from build123d import *

# Parameters (mm, degrees)
SKETCH1_R           = 2.5
SKETCH1_R_2         = 10.25
BOSS_EXTRUDE1_DEPTH = 5


with BuildPart() as part:
    # Sketch1 → Boss-Extrude1 (new body)
    with BuildSketch(Plane.XY):
        with BuildLine():
            Line((-18.262940366, -7.217732658), (-10.073546599, -13.382307683))
            ThreePointArc((-10.073546599, -13.382307683), (0, -16.75), (10.073546599, -13.382307683))
            Line((10.073546599, -13.382307683), (18.262940366, -7.217732658))
            ThreePointArc((18.262940366, -7.217732658), (21.863878029, 0), (18.262940366, 7.217732658))
            Line((18.262940366, 7.217732658), (10.073546599, 13.382307683))
            ThreePointArc((10.073546599, 13.382307683), (0, 16.75), (-10.073546599, 13.382307683))
            Line((-10.073546599, 13.382307683), (-18.262940366, 7.217732658))
            ThreePointArc((-18.262940366, 7.217732658), (-21.863878029, 0), (-18.262940366, -7.217732658))
        make_face()
        with Locations((14.5, 0)):
            Circle(SKETCH1_R, mode=Mode.SUBTRACT)
        with Locations((-14.5, 0)):
            Circle(SKETCH1_R, mode=Mode.SUBTRACT)
        Circle(SKETCH1_R_2, mode=Mode.SUBTRACT)
    extrude(amount=BOSS_EXTRUDE1_DEPTH)


solid = part.part
Verification items for the finished model (mm, model axes). Coordinates: 2 decimals unless noted, no trailing zeros. Write each loop counter-clockwise with the first axis right and the second up, starting at its lowest first coordinate (ties: lowest second). Pieces come first, ordered by that corner, then holes. Notation, with made-up numbers: (81, 15.5) - (140, 15.5) arc R23 cw to (140, 54.5) - close; hole circle Ø10 at (82, 37). An arc over 180 degrees is marked (long way). Answer as a JSON object with one key per item and string values.
(1) Cross-section at A-A on x = 0. Record the cut outline in (y, z), plus the area to 3 significant figures.
Report:
{"outline": "(-16.75, 0) - (-10.25, 0) - (-10.25, 5) - (-16.75, 5) - close; (10.25, 0) - (16.75, 0) - (16.75, 5) - (10.25, 5) - close", "area": "65.0 mm^2"}
(2) Cross-section at B-B on y = 0. Record the cut outline in (x, z), plus the area to 3 significant figures.
Report:
{"outline": "(-21.86, 0) - (-17, 0) - (-17, 5) - (-21.86, 5) - close; (-12, 0) - (-10.25, 0) - (-10.25, 5) - (-12, 5) - close; (10.25, 0) - (12, 0) - (12, 5) - (10.25, 5) - close; (17, 0) - (21.86, 0) - (21.86, 5) - (17, 5) - close", "area": "66.1 mm^2"}
(3) Cross-section at C-C on z = 3.5. Record the cut outline in (x, y).
Report:
{"outline": "(-18.26, -7.22) - (-10.07, -13.38) arc R16.75 ccw to (10.07, -13.38) - (18.26, -7.22) arc R9.03 ccw to (18.26, 7.22) - (10.07, 13.38) arc R16.75 ccw to (-10.07, 13.38) - (-18.26, 7.22) arc R9.03 ccw to start; hole circle Ø5 at (-14.5, 0); hole circle Ø20.5 at (0, 0); hole circle Ø5 at (14.5, 0)"}
(4) Thickness scan on line 1 along Y through (x, z) = (-7, 0.45); line 2 along Y through (x, z) = (-14.5, 1.95); line 3 along X through (y, z) = (-11.5, 0.45). Record the ranges inside material, lowest first.
Report:
{"line 1": "-15.22 to -7.49, 7.49 to 15.22", "line 2": "-10.05 to -2.5, 2.5 to 10.05", "line 3": "-12.57 to 12.57"}
(5) Gauge pin test, flat ends, axial feed: pin 1 Ø18.5 at (x, y) = (0, 0) entering from +Z; pin 2 Ø3 at (y, z) = (13, 3.5) entering from +X. Record the tip position at first contact, or that the pin passes through.
Report:
{"pin 1": "through", "pin 2": "x = 12.57"}
(6) Mould release check, pull along Y, two halves, no side actions. Record for faces 1 (the cylindrical face through (-17, 0, 2)), 2 (the flat face through (14.111, -10.343, 2.465)), 3 (the cylindrical face through (-2.222, -10.006, 2.465)), 4 (the cylindrical face through (-21.863, 0.117, 2.465)): pulls with the +Y half, pulls with the -Y half, needs draft (parallel to the pull), parting line crosses it, or undercut.
Report:
{"face 1": "undercut", "face 2": "pulls with the -Y half", "face 3": "undercut", "face 4": "parting line crosses it"}
(7) Cross-section at D-D on x = -7. Record the cut outline in (y, z), plus the area to 3 significant figures.
Report:
{"outline": "(-15.22, 0) - (-7.49, 0) - (-7.49, 5) - (-15.22, 5) - close; (7.49, 0) - (15.22, 0) - (15.22, 5) - (7.49, 5) - close", "area": "77.3 mm^2"}
